```python
from build123d import *

# Parameters (mm, degrees)
F0_W     = 542.925
F0_H     = 292.1
F1_DEPTH = 19.05
F2_W     = 254
F2_H     = 203.2
F3_DEPTH = 6.35
F4_R     = 12.7
F5_R     = 77.7875
F6_DEPTH = 12.7


with BuildPart() as f1:
    # F0 (on Top) → F1 (new body)
    with BuildSketch(Plane.XY):
        Rectangle(F0_W, F0_H)
    extrude(amount=F1_DEPTH)

    # F2 (on face) → F3 (cut)
    with BuildSketch(Plane.XY.offset(19.05)):
        Rectangle(F2_W, F2_H)
    extrude(amount=-F3_DEPTH, mode=Mode.SUBTRACT)

    # F4
    f4_edges = [f1.edges().sort_by_distance(p)[0] for p in [
        (127, -101.6, 15.875),
        (-127, -101.6, 15.875),
        (-127, 101.6, 15.875),
        (127, 101.6, 15.875),
    ]]
    fillet(f4_edges, radius=F4_R)

    # F5 (on face) → F6 (cut, through all)
    with BuildSketch(Plane.XY.offset(12.7)):
        Circle(F5_R)
    extrude(amount=-F6_DEPTH, mode=Mode.SUBTRACT)


solid = f1.part
```
The model under review builds one solid part; all positions refer to its coordinate system, in mm. A direction names the side the tool comes from. Give positions to 0.01 mm unless a question says otherwise; leave off trailing zeros. Write each loop counter-clockwise with the first axis right and the second up, starting at its lowest first coordinate (ties: lowest second). Pieces come first, ordered by that corner, then holes. Notation, with made-up numbers: M -2.75,-11 L 29.25,-11 A17 cw 29.25,4 Z; hole C -33,27 d6. An arc over 180 degrees is marked long. Answer in a Markdown table with one row per item.
Item 1: Add section A-A on x = 0. Give the boundary of the cut face in (y, z), plus the area to 3 significant figures.
Check sheet entries:
| item | result |
|---|---|
| outline | M -146.05,0 L -77.79,0 L -77.79,12.7 L -101.6,12.7 L -101.6,19.05 L -146.05,19.05 Z; M 77.79,0 L 146.05,0 L 146.05,19.05 L 101.6,19.05 L 101.6,12.7 L 77.79,12.7 Z |
| area | 2,300 mm2 |
Item 2: For line 1 along Y through (x, z) = (0, 9); line 2 along Y through (x, z) = (61, 15.25); line 3 along Z through (x, y) = (92, -34), list the stretches that pass through material, from the lowest coordinate up.
Check sheet entries:
| item | result |
|---|---|
| line 1 | -146.05 to -77.79, 77.79 to 146.05 |
| line 2 | -146.05 to -101.6, 101.6 to 146.05 |
| line 3 | 0 to 12.7 |
Item 3: Add section D-D on x = -102. Give the boundary of the cut face in (y, z), plus the area to 3 significant figures.
Check sheet entries:
| item | result |
|---|---|
| outline | M -146.05,0 L 146.05,0 L 146.05,19.05 L 101.6,19.05 L 101.6,12.7 L -101.6,12.7 L -101.6,19.05 L -146.05,19.05 Z |
| area | 4,270 mm2 |
Item 4: Draft analysis for pull direction Y (two halves, no side actions). For faces 1 (the face through (-123.18, -97.98, 15.83)), 2 (the face through (-64, 67, 0)), 3 (the face through (-61.73, -47.33, 6.44)), 4 (the face through (-4, 146.05, 9)), state which applies: +Y half, -Y half, draft (parallel to the pull), parting line (faces both ways), or undercut.
Check sheet entries:
| item | result |
|---|---|
| face 1 | undercut |
| face 2 | draft |
| face 3 | undercut |
| face 4 | +Y half |
Item 5: Add section B-B on y = 0. Give the boundary of the cut face in (x, z), plus the area to 3 significant figures.
Check sheet entries:
| item | result |
|---|---|
| outline | M -271.46,0 L -77.79,0 L -77.79,12.7 L -127,12.7 L -127,19.05 L -271.46,19.05 Z; M 77.79,0 L 271.46,0 L 271.46,19.05 L 127,19.05 L 127,12.7 L 77.79,12.7 Z |
| area | 6,750 mm2 |
Item 6: Tool access review of faces 5 (the face through (123.18, -97.98, 15.83)), 6 (the face through (-4, 132, 19.05)): name each direction out of +Z, -Z, +X, -X, +Y, -Y from which nothing blocks a thin tool from reaching the whole face with its end or side.
Check sheet entries:
| item | result |
|---|---|
| face 5 | +Z |
| face 6 | +Z, +X, -X, +Y, -Y |
